Autodesk Inventor part; units mm, degrees
ref_plane "YZ Plane" through (0, 0, 0) normal (1, 0, 0) x (0, 1, 0)
ref_plane "XZ Plane" through (0, 0, 0) normal (0, 1, 0) x (-1, 0, 0)
ref_plane "XY Plane" through (0, 0, 0) normal (0, 0, 1) x (1, 0, 0)
sketch "Sketch1" plane through (0, 0, 0) normal (0, 0, 1) x (1, 0, 0)
  line L0 (-14, 0) -> (14, 0)
  line L1 (14, 0) -> (14, 75)
  line L2 (14, 75) -> (-14, 75)
  line L3 (-14, 75) -> (-14, 0)
  circle A0 centre (-9, 5) radius 1.75
  circle A1 centre (9, 5) radius 1.75
  line L4 (-9, 5) -> (9, 5)
  point P0 (0, 0)
  point P1 (0, 0)
  point P2 (0, 5)
  dimension "d0" = 75
  dimension "d2" = 28
  dimension "d3" = 5
  dimension "d4" = 3.5
  dimension "d5" = 18
extrude "Extrusion1" add sketch "Sketch1" along normal blind 2
sketch "Sketch4" plane through (0, 0, 2) normal (0, 0, 1) x (1, 0, 0)
  line L0 (14, 75) -> (-14, 75)
  line L1 (-10.5, 70) -> (10.5, 70)
  line L2 (10.5, 70) -> (10.5, 68)
  line L3 (10.5, 68) -> (-10.5, 68)
  line L4 (-10.5, 68) -> (-10.5, 70)
  line L5 (-10.5, 53) -> (10.5, 53)
  line L6 (10.5, 53) -> (10.5, 55)
  line L7 (10.5, 55) -> (-10.5, 55)
  line L8 (-10.5, 55) -> (-10.5, 53)
  point P0 (0, 0)
  point P1 (0, 53)
  point P2 (0, 68)
  point P3 (0, 75)
  dimension "d19" = 21
  dimension "d21" = 2
  dimension "d22" = 5
  dimension "d23" = 15
extrude "Extrusion4" cut sketch "Sketch4" against normal through all
fillet "Fillet2" radius 5 4 edges at (14, 75, 1) (-14, 75, 1) (14, 0, 1) (-14, 0, 1)
sketch "Sketch2" plane through (0, 0, 2) normal (0, 0, 1) x (1, 0, 0)
  line L0 (14, 75) -> (-14, 75)
  line L1 (-11, 75) -> (11, 75)
  line L2 (11, 75) -> (11, 65)
  line L3 (11, 65) -> (-11, 65)
  line L4 (-11, 65) -> (-11, 75)
  line L5 (-11, 65) -> (-14, 65)
  line L6 (-14, 65) -> (-14, 75)
  line L7 (-14, 75) -> (-11, 75)
  line L8 (-11, 75) -> (-11, 65)
  line L9 (11, 65) -> (14, 65)
  line L10 (14, 65) -> (14, 75)
  line L11 (14, 75) -> (11, 75)
  line L12 (11, 75) -> (11, 65)
  point P0 (0, 0)
  point P1 (0, 75)
  dimension "d8" = 10
  dimension "d10" = 22
sketch "Sketch3" plane through (0, 0, 4) normal (0, 0, 1) x (1, 0, 0)
  line L0 (-11, 65) -> (-11, 75)
  line L1 (-11, 75) -> (-14, 75)
  line L2 (-14, 75) -> (-14, 65)
  line L3 (-14, 65) -> (-11, 65)
  line L4 (14, 75) -> (11, 75)
  line L5 (11, 75) -> (11, 65)
  line L6 (11, 65) -> (14, 65)
  line L7 (14, 65) -> (14, 75)
  line L8 (-11, 75) -> (11, 75)
  line L9 (11, 75) -> (11, 65)
  line L10 (11, 65) -> (-11, 65)
  line L11 (-11, 65) -> (-11, 75)
  point P0 (0, 0)
properties part number "ribbon slider manager"
Geometry: final body of the model. Coordinates: model frame, mm. A direction names the side the tool comes from. Give positions to 0.01 mm unless a question says otherwise; leave off trailing zeros. Write each loop counter-clockwise with the first axis right and the second up, starting at its lowest first coordinate (ties: lowest second). Pieces come first, ordered by that corner, then holes. Notation, with made-up numbers: M 81,56.5 L 131,56.5 A5 ccw 131,62.5 Z; hole C 83,55 d11. An arc over 180 degrees is marked long. Answer in a Markdown table with one row per item. Add a question column.
(1) Ray query, line 1 (Y direction, x = 9, z = 1.2); line 2 (Y direction, x = 6.75, z = 0.7); line 3 (Y direction, x = -9.75, z = 1.3). Return the intervals inside material, ascending.
(2) First-contact query: pin 1 (2 mm diameter, centred on x = 9, y = 5, fed in from -Z). Flat tip, straight axial feed; report the tip coordinate or a pass-through.
(3) Mould query, pull axis X, two halves, no side actions, for faces 3 (the cylindrical face through (10.617, 5.67, 0.986)), 4 (the cylindrical face through (-13, 2, 1)), 5 (the flat face through (0, 75, 1)). Classes: +X half, -X half, draft (parallel to the pull), parting line (faces both ways), or undercut.
(4) Section A-A on z = 0.85. Return loops of the section in (x, y), and give its area (3 significant figures).
(5) Reachability of faces 1 (the flat face through (10.5, 54, 1)), 2 (the cylindrical face through (12, 1, 1)) from +Z, -Z, +X, -X, +Y, -Y: full face, straight path, thin tool, end or side. Return the list, or none.
Result set:
| question | item | result |
|---|---|---|
| 1 | line 1 | y = 0 to 3.25, 6.75 to 53, 55 to 68, 70 to 75 |
| 1 | line 2 | y = 0 to 53, 55 to 68, 70 to 75 |
| 1 | line 3 | y = 0.06 to 3.42, 6.58 to 53, 55 to 68, 70 to 74.94 |
| 2 | pin 1 | passes through |
| 3 | face 3 | undercut |
| 3 | face 4 | -X half |
| 3 | face 5 | draft |
| 4 | outline | M -14,5 A5 ccw -9,0 L 9,0 A5 ccw 14,5 L 14,70 A5 ccw 9,75 L -9,75 A5 ccw -14,70 Z; hole C -9,5 d3.5; hole M -10.5,53 L 10.5,53 L 10.5,55 L -10.5,55 Z; hole M -10.5,68 L 10.5,68 L 10.5,70 L -10.5,70 Z; hole C 9,5 d3.5 |
| 4 | area | 1,980 mm^2 |
| 5 | face 1 | +Z, -Z |
| 5 | face 2 | +Z, -Z, +X, -Y |
